```python
from build123d import *

# Parameters (mm, degrees)
SKETCH1_R           = 4.8
SKETCH1_R_2         = 12.7
BOSS_EXTRUDE1_DEPTH = 5.45
CHAMFER1_SIZE       = 0.8


with BuildPart() as part:
    # Sketch1 → Boss-Extrude1 (new, symmetric)
    with BuildSketch(Plane(origin=(0, 0, 0), x_dir=(1, 0, 0), z_dir=(0, 1, 0))):
        with BuildLine():
            Line((-37.865350224, 11.944360697), (-8.188971684, 22.666070298))
            ThreePointArc((-8.188971684, 22.666070298), (0, 24.1), (8.188971684, 22.666070298))
            Line((8.188971684, 22.666070298), (37.865350224, 11.944360697))
            ThreePointArc((37.865350224, 11.944360697), (46.25, 0), (37.865350224, -11.944360697))
            Line((37.865350224, -11.944360697), (8.188971684, -22.666070298))
            ThreePointArc((8.188971684, -22.666070298), (0, -24.1), (-8.188971684, -22.666070298))
            Line((-8.188971684, -22.666070298), (-37.865350224, -11.944360697))
            ThreePointArc((-37.865350224, -11.944360697), (-46.25, 0), (-37.865350224, 11.944360697))
        make_face()
        with Locations(Location((-33.55, 0, 0), (0, 0, 270))):
            Circle(SKETCH1_R, mode=Mode.SUBTRACT)
        with Locations(Location((33.55, 0, 0), (0, 0, 270))):
            Circle(SKETCH1_R, mode=Mode.SUBTRACT)
        with Locations(Location((0, 0, 0), (0, 0, 270))):
            Circle(SKETCH1_R_2, mode=Mode.SUBTRACT)
    extrude(amount=BOSS_EXTRUDE1_DEPTH, both=True)

    # Chamfer1
    chamfer1_edges = [part.edges().sort_by_distance(p)[0] for p in [
        (-33.55, -5.45, -4.8),
        (-33.55, 5.45, -4.8),
        (33.55, -5.45, -4.8),
        (33.55, 5.45, -4.8),
        (0, -5.45, -12.7),
        (0, 5.45, -12.7),
    ]]
    chamfer(chamfer1_edges, length=CHAMFER1_SIZE)


solid = part.part
```
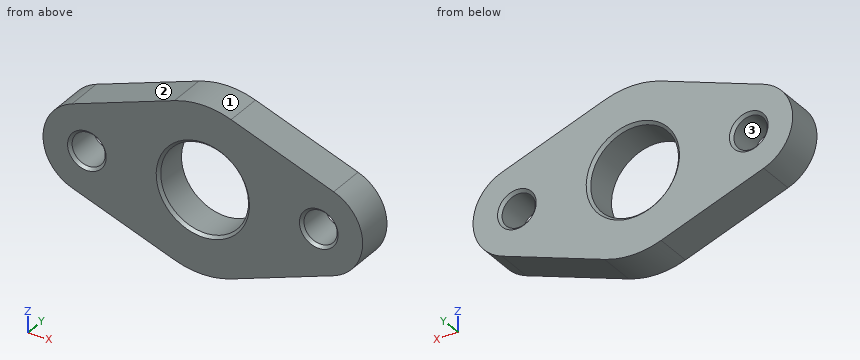
Build history of the part. All positions in model axes, mm. Face numbers are marked on the shaded views. Round coordinates to 2 decimals unless told otherwise and drop trailing zeros. Order: outer loops, then holes, each group sorted by start corner. A loop starts at its lowest first (then second) coordinate and runs counter-clockwise, first axis right, second up. Notation, with made-up numbers: (44, 39.25) -> (85, 39.25) arc R23 ccw to (85, 53.25) -> close; hole circle Ø9 at (82, -26). An arc over 180 degrees is marked (long way). Answer in a Markdown table with one row per item.
1) Mould opens along X. For the marked faces 1, 2 and 3 say: released by +X, released by -X, zero draft, split by the parting line, or undercut.
Values:
| item | result |
|---|---|
| face 1 | split by the parting line |
| face 2 | released by -X |
| face 3 | undercut |
2) Pin check, flat tips, straight feed: P1, Ø8.5, axis at x = 33.55, z = 0, coming from the -Y side; P2, Ø3, axis at y = -2.5, z = -9.5, coming from the -X side; P3, Ø1, axis at x = -19, y = -3.5, coming from the -Z side. Stop position of each tip, or through.
Values:
| item | result |
|---|---|
| P1 | through |
| P2 | x = -43.41 |
| P3 | z = -18.94 |
3) Band-saw the part on B-B on y = 3. Give the cut face in (x, z).
Values:
| item | result |
|---|---|
| outline | (-37.87, -11.94) -> (-8.19, -22.67) arc R24.1 ccw to (8.19, -22.67) -> (37.87, -11.94) arc R12.7 ccw to (37.87, 11.94) -> (8.19, 22.67) arc R24.1 ccw to (-8.19, 22.67) -> (-37.87, 11.94) arc R12.7 ccw to start; hole circle Ø9.6 at (-33.55, 0); hole circle Ø25.4 at (0, 0); hole circle Ø9.6 at (33.55, 0) |
4) Band-saw the part on D-D on x = 0. Give the cut face in (y, z).
Values:
| item | result |
|---|---|
| outline | (-5.45, -24.1) -> (5.45, -24.1) -> (5.45, -13.5) -> (4.65, -12.7) -> (-4.65, -12.7) -> (-5.45, -13.5) -> close; (-5.45, 13.5) -> (-4.65, 12.7) -> (4.65, 12.7) -> (5.45, 13.5) -> (5.45, 24.1) -> (-5.45, 24.1) -> close |
5) Band-saw the part on C-C on x = 33.55. Give the cut face in (y, z), and give its area (3 significant figures).
Values:
| item | result |
|---|---|
| outline | (-5.45, -13.5) -> (5.45, -13.5) -> (5.45, -5.6) -> (4.65, -4.8) -> (-4.65, -4.8) -> (-5.45, -5.6) -> close; (-5.45, 5.6) -> (-4.65, 4.8) -> (4.65, 4.8) -> (5.45, 5.6) -> (5.45, 13.5) -> (-5.45, 13.5) -> close |
| area | 188 mm2 |
6) Band-saw the part on A-A on z = 0. Give the cut face in (x, y).
Values:
| item | result |
|---|---|
| outline | (-46.25, -5.45) -> (-39.15, -5.45) -> (-38.35, -4.65) -> (-38.35, 4.65) -> (-39.15, 5.45) -> (-46.25, 5.45) -> close; (-28.75, -4.65) -> (-27.95, -5.45) -> (-13.5, -5.45) -> (-12.7, -4.65) -> (-12.7, 4.65) -> (-13.5, 5.45) -> (-27.95, 5.45) -> (-28.75, 4.65) -> close; (12.7, -4.65) -> (13.5, -5.45) -> (27.95, -5.45) -> (28.75, -4.65) -> (28.75, 4.65) -> (27.95, 5.45) -> (13.5, 5.45) -> (12.7, 4.65) -> close; (38.35, -4.65) -> (39.15, -5.45) -> (46.25, -5.45) -> (46.25, 5.45) -> (39.15, 5.45) -> (38.35, 4.65) -> close |
7) Wall check: L1, parallel to X at y = -0.75, z = 3; L2, parallel to Z at x = 31.5, y = -4.25; L3, parallel to X at y = -2, z = 10. Give the ranges that are in metal, low to high.
Values:
| item | result |
|---|---|
| L1 | -45.89 to -37.3, -29.8 to -12.34, 12.34 to 29.8, 37.3 to 45.89 |
| L2 | -14.24 to -4.34, 4.34 to 14.24 |
| L3 | -41.38 to -7.83, 7.83 to 41.38 |
